Geometry: final body of the model. Coordinates: model frame, mm. Give positions to 0.01 mm unless a question says otherwise; leave off trailing zeros. Write each loop counter-clockwise with the first axis right and the second up, starting at its lowest first coordinate (ties: lowest second). Pieces come first, ordered by that corner, then holes. Notation, with made-up numbers: (-1.75, -37.5) - (22.25, -37.5) arc R33 ccw to (22.25, 0.5) - close; hole circle Ø1 at (10, 55.5). An arc over 180 degrees is marked (long way). One line per question, with ' | ' between items. Start each with the question number.
Autodesk Inventor part; units mm, degrees
ref_plane "YZ Plane" through (0, 0, 0) normal (1, 0, 0) x (0, 1, 0)
ref_plane "XZ Plane" through (0, 0, 0) normal (0, 1, 0) x (-1, 0, 0)
ref_plane "XY Plane" through (0, 0, 0) normal (0, 0, 1) x (1, 0, 0)
sketch "Boceto1" plane through (0, 0, 0) normal (0, 1, 0) x (-1, 0, 0)
  line L0 (0, 0) -> (-105, 0)
  line L1 (-105, 0) -> (-105, -140)
  line L2 (-105, -140) -> (0, -140)
  line L3 (0, -140) -> (0, 0)
  dimension "d0" = 105
  dimension "d1" = 140
extrude "Extrusión1" add sketch "Boceto1" along normal blind 3
sketch "Boceto2" plane through (0, 3, 0) normal (0, 1, 0) x (1, 0, 0)
  line L0 (0, 0) -> (105, 0)
  line L1 (105, 0) -> (105, 140)
  line L2 (105, 140) -> (0, 140)
  line L3 (0, 140) -> (0, 0)
  circle A0 centre (52.5, 46) radius 38.5
  circle A1 centre (52.5, 111) radius 18
  dimension "d4" = 77
  dimension "d5" = 46
  dimension "d6" = 52.5
  dimension "d7" = 36
  dimension "d8" = 52.5
  dimension "d13" = 65
extrude "Extrusión2" cut sketch "Boceto2" against normal blind 3 contours A0 | A1
sketch "Boceto3" plane through (0, 0, 0) normal (0, -1, 0) x (1, 0, 0)
  circle A0 centre (52.5, -111) radius 18
  circle A1 centre (52.5, -46) radius 38.5
  line L0 (0, 0) -> (105, 0)
  line L1 (0, -140) -> (0, 0)
  line L2 (105, -140) -> (0, -140)
  line L3 (105, 0) -> (105, -140)
  line L4 (105, -140) -> (0, -140)
  line L5 (0, -140) -> (0, 0)
  line L6 (105, -140) -> (0, -140)
  line L7 (0, -140) -> (0, -136)
  line L8 (0, -136) -> (105, -136)
  line L9 (105, -136) -> (105, -140)
  dimension "d14" = 4
extrude "Extrusión3" cut sketch "Boceto3" against normal blind 3 contours L8 L3 L2 L1
sketch "Boceto4" plane through (0, 0, 0) normal (0, -1, 0) x (1, 0, 0)
  line L0 (0, -136) -> (105, -136)
  line L1 (105, 0) -> (105, -136)
  line L2 (0, 0) -> (105, 0)
  line L3 (0, -136) -> (0, 0)
  circle A0 centre (52.5, -111) radius 18
  circle A1 centre (52.5, -46) radius 38.5
  line L4 (105, -136) -> (0, -136)
  line L5 (2.5, 0) -> (102.5, 0)
  line L6 (102.5, 0) -> (102.5, -136)
  line L7 (102.5, -136) -> (2.5, -136)
  line L8 (2.5, -136) -> (2.5, 0)
  line L9 (2.5, 0) -> (102.5, -136) construction
  line L10 (102.5, 0) -> (2.5, -136) construction
  point P0 (52.5, -68)
  dimension "d17" = 100
extrude "Extrusión4" cut sketch "Boceto4" against normal blind 3 contours L3 L2 L8 L0 | L6 L2 L1 L0
sketch "Boceto5" plane through (0, 3, 0) normal (0, 1, 0) x (1, 0, 0)
  point P0 (0, 0)
sketch "Boceto6" plane through (2.5, 0, 0) normal (0, 0, 1) x (1, 0, 0)
  line L0 (0, 3) -> (0, 0)
  line L1 (0, 0) -> (100, 0)
  line L2 (100, 0) -> (100, 3)
  line L3 (0, 3) -> (100, 3)
  point P0 (-2.5, 0)
extrude "Extrusión5" cut sketch "Boceto6" against normal blind 1
sketch "Boceto7" plane through (0, 3, 0) normal (0, 1, 0) x (1, 0, 0)
  line L0 (2.5, 1) -> (102.5, 1)
  line L1 (102.5, 1) -> (102.5, 136)
  line L2 (102.5, 136) -> (2.5, 136)
  line L3 (2.5, 136) -> (2.5, 1)
  circle A0 centre (52.5, 46) radius 38.5
  circle A1 centre (52.5, 111) radius 18
  line L4 (102.5, 136) -> (2.5, 136)
  line L5 (100, 1) -> (5, 1)
  line L6 (5, 1) -> (5, 136)
  line L7 (5, 136) -> (100, 136)
  line L8 (100, 136) -> (100, 1)
  line L9 (100, 1) -> (5, 136) construction
  line L10 (5, 1) -> (100, 136) construction
  point P0 (0, 0)
  point P1 (52.5, 68.5)
  dimension "d22" = 95
extrude "Extrusión6" cut sketch "Boceto7" against normal blind 3 contours L3 L2 L6 L0 | L8 L2 L1 L0
equation "\"d8\" = d6"
properties part number "frontal"
1) First-contact query: pin 1 Ø5 at (x, z) = (22.5, -77.5) entering from -Y; pin 2 Ø21.5 at (x, z) = (52.5, -111) entering from -Y. Flat tips, straight axial feed; report the tip coordinate or a pass-through.
2) Section C-C, the plane y = 2.4. Output: boundary loops of the cut face in (x, z), plus the area to 3 significant figures.
3) Line query: L1, parallel to Z at x = 52.5, y = 1.45; L2, parallel to X at y = 1.55, z = -111; L3, parallel to Z at x = 37, y = 2.65. Output: solid intervals per line, ascending.
4) Section B-B, the plane z = -46. Output: boundary loops of the cut face in (x, y).
5) Section A-A, the plane x = 52.5. Output: boundary loops of the cut face in (y, z).
6) Section D-D, the plane z = -111. Output: boundary loops of the cut face in (x, y).
7) Pull-direction query (X, two-part tool) for faces 1 (the flat face through (100, 2, -69)), 2 (the flat face through (5, 2, -68)), 3 (the cylindrical face through (69.669, 1.521, -116.407)); classes: +X half, -X half, draft (parallel to the pull), parting line (faces both ways), or undercut.
Answer key:
1) pin 1: y = 0 | pin 2: through
2) outline: (5, -136) - (100, -136) - (100, -1) - (5, -1) - close; hole circle Ø77 at (52.5, -46); hole circle Ø36 at (52.5, -111) | area: 7,150 mm^2
3) L1: -136 to -129, -93 to -84.5, -7.5 to -1 | L2: 5 to 34.5, 70.5 to 100 | L3: -136 to -120.15, -101.85 to -81.24, -10.76 to -1
4) outline: (5, 0) - (14, 0) - (14, 3) - (5, 3) - close; (91, 0) - (100, 0) - (100, 3) - (91, 3) - close
5) outline: (0, -136) - (3, -136) - (3, -129) - (0, -129) - close; (0, -93) - (3, -93) - (3, -84.5) - (0, -84.5) - close; (0, -7.5) - (3, -7.5) - (3, -1) - (0, -1) - close
6) outline: (5, 0) - (34.5, 0) - (34.5, 3) - (5, 3) - close; (70.5, 0) - (100, 0) - (100, 3) - (70.5, 3) - close
7) face 1: +X half | face 2: -X half | face 3: undercut
